Part model, mm, in its own coordinate system. Face numbers are marked on the shaded views. A direction names the side the tool comes from. Give positions to 0.01 mm unless a question says otherwise; leave off trailing zeros. Write each loop counter-clockwise with the first axis right and the second up, starting at its lowest first coordinate (ties: lowest second). Pieces come first, ordered by that corner, then holes. Notation, with made-up numbers: M 35,8 L 81,8 A8 cw 81,16 Z; hole C 54,83 d11. An arc over 180 degrees is marked long. Use a Markdown table: item, result.
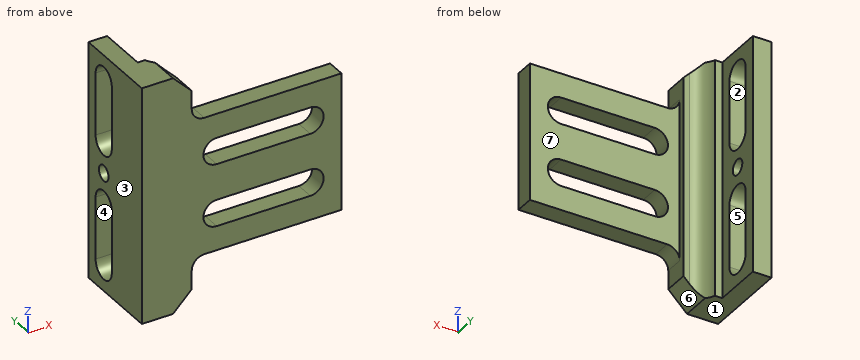
```python
from build123d import *

# Parameters (mm, degrees)
BASESTEELANGLE_DEPTH    = 60.325
CUT_EXTRUDE1_DEPTH      = 1
CUT_EXTRUDE1_DEPTH_BACK = 121.65
CUT_EXTRUDE3_DEPTH      = 13.7
SKETCH5_W               = 76.2
SKETCH5_H               = 6.35
CUT_EXTRUDE4_DEPTH      = 121.65
SKETCH6_W               = 9.525
SKETCH6_H               = 28.575
CUT_EXTRUDE5_DEPTH      = 121.65
CUT_EXTRUDE6_DEPTH      = 10.525
F_3_8_16_TAPPED_HOLE1_D = 7.9375
SKETCH11_W              = 25.4
SKETCH11_H              = 9.525
CUT_EXTRUDE8_DEPTH      = 76.2
FILLET2_R               = 6.35
CHAMFER3_SIZE           = 9.525


with BuildPart() as part:
    # Sketch1 → BaseSteelAngle (new body, symmetric)
    with BuildSketch(Plane.XY):
        with BuildLine():
            Line((0, 0), (0, 101.6))
            Line((0, 101.6), (3.18008, 101.6))
            ThreePointArc((3.18008, 101.6), (9.911679988, 98.811679988), (12.7, 92.08008))
            Line((12.7, 92.08008), (12.7, 22.225))
            ThreePointArc((12.7, 22.225), (15.489807909, 15.489807909), (22.225, 12.7))
            Line((22.225, 12.7), (101.6, 12.7))
            Line((101.6, 12.7), (101.6, 0))
            Line((101.6, 0), (0, 0))
        make_face()
    extrude(amount=BASESTEELANGLE_DEPTH, both=True)

    # Sketch2 → Cut-Extrude1 (cut, two sides)
    with BuildSketch(Plane.XY.offset(60.325)) as cut_extrude1_sk:
        Polygon((-254.455417258, 44.45), (-4.112271749, 44.45), (18.408340367, 44.45), (268.751485876, 44.45), (268.751485876, 545.136291018), (-254.455417258, 545.136291018), align=None)
    extrude(amount=CUT_EXTRUDE1_DEPTH, mode=Mode.SUBTRACT)
    extrude(cut_extrude1_sk.sketch, amount=-CUT_EXTRUDE1_DEPTH_BACK, mode=Mode.SUBTRACT)

    # Sketch4 → Cut-Extrude3 (cut, through all)
    with BuildSketch(Plane(origin=(78.166939161, 12.7, 45.281727152), x_dir=(0, 0, 1), z_dir=(0, 1, 0))):
        with BuildLine():
            Line((-67.902967152, 7.558060839), (-67.902967152, -40.066939161))
            ThreePointArc((-67.902967152, -40.066939161), (-61.156727152, -46.813179161), (-54.410487152, -40.066939161))
            Line((-54.410487152, -40.066939161), (-54.410487152, 7.558060839))
            ThreePointArc((-54.410487152, 7.558060839), (-61.156727152, 14.304300839), (-67.902967152, 7.558060839))
        make_face()
    cut_extrude3 = extrude(amount=-CUT_EXTRUDE3_DEPTH, mode=Mode.SUBTRACT)

    # Mirror1: Cut-Extrude3 across plane
    add(cut_extrude3.mirror(Plane.XY), mode=Mode.SUBTRACT)

    # Sketch5 → Cut-Extrude4 (cut, through all)
    with BuildSketch(Plane(origin=(0, 0, -60.325), x_dir=(-1, 0, 0), z_dir=(0, 0, -1))):
        with Locations((-63.5, 12.7)):
            Rectangle(SKETCH5_W, SKETCH5_H)
    extrude(amount=-CUT_EXTRUDE4_DEPTH, mode=Mode.SUBTRACT)

    # Sketch6 → Cut-Extrude5 (cut, through all)
    with BuildSketch(Plane(origin=(0, 0, -60.325), x_dir=(-1, 0, 0), z_dir=(0, 0, -1))):
        with Locations((-14.2875, 33.3375)):
            Rectangle(SKETCH6_W, SKETCH6_H)
    extrude(amount=-CUT_EXTRUDE5_DEPTH, mode=Mode.SUBTRACT)

    # Sketch7 → Cut-Extrude6 (cut, through all)
    with BuildSketch(Plane(origin=(9.525, 0, 0), x_dir=(0, 0, -1), z_dir=(1, 0, 0))):
        with BuildLine():
            Line((15.875, 25.003125), (47.625, 25.003125))
            ThreePointArc((47.625, 25.003125), (54.371875, 31.75), (47.625, 38.496875))
            Line((47.625, 38.496875), (15.875, 38.496875))
            ThreePointArc((15.875, 38.496875), (9.128125, 31.75), (15.875, 25.003125))
        make_face()
    cut_extrude6 = extrude(amount=-CUT_EXTRUDE6_DEPTH, mode=Mode.SUBTRACT)

    # Mirror2: Cut-Extrude6 across plane
    add(cut_extrude6.mirror(Plane.XY), mode=Mode.SUBTRACT)

    # 3/8-16 Tapped Hole1 (through all)
    with Locations(Plane(origin=(9.525, 0, 0), x_dir=(0, 0, -1), z_dir=(1, 0, 0))):
        with Locations((0, 31.75)):
            Hole(F_3_8_16_TAPPED_HOLE1_D / 2)

    # Sketch11 → Cut-Extrude8 (cut)
    with BuildSketch(Plane(origin=(101.6, 0, 0), x_dir=(0, 0, -1), z_dir=(1, 0, 0))):
        with Locations((47.625, 4.7625)):
            Rectangle(SKETCH11_W, SKETCH11_H)
        with Locations((-47.625, 4.7625)):
            Rectangle(SKETCH11_W, SKETCH11_H)
    extrude(amount=-CUT_EXTRUDE8_DEPTH, mode=Mode.SUBTRACT)

    # Fillet2
    fillet2_edges = [part.edges().sort_by_distance(p)[0] for p in [
        (25.4, 4.7625, -34.925),
        (25.4, 4.7625, 34.925),
    ]]
    fillet(fillet2_edges, radius=FILLET2_R)

    # Chamfer3
    chamfer3_edges = [part.edges().sort_by_distance(p)[0] for p in [
        (25.4, 6.35, 60.325),
        (25.4, 6.35, -60.325),
    ]]
    chamfer(chamfer3_edges, length=CHAMFER3_SIZE)


solid = part.part
```
1. Drill centre lines: L1, parallel to Z at x = 79, y = 7.5 (3 decimals); L2, parallel to Y at x = 3, z = 0; L3, parallel to Y at x = 8.5, z = 32.5. Where is each one in solid material? Low to high.
Findings below:
| item | result |
|---|---|
| L1 | -34.925 to -22.621, -9.129 to 9.129, 22.621 to 34.925 |
| L2 | 0 to 27.78, 35.72 to 44.45 |
| L3 | 0 to 25, 38.5 to 44.45 |
2. Cut at D-D, the plane z = 21. Give the cut face in (x, y) (3 decimals).
Findings below:
| item | result |
|---|---|
| outline | M 0,0 L 33.713,0 L 33.713,9.525 L 25.4,9.525 L 25.4,12.7 L 22.225,12.7 A9.525 cw 13.245,19.05 L 9.525,19.05 L 9.525,25.003 L 0,25.003 Z; M 0,38.497 L 9.525,38.497 L 9.525,44.45 L 0,44.45 Z; M 90.112,0 L 101.6,0 L 101.6,9.525 L 90.112,9.525 Z |
3. Cut at C-C, the plane y = 31.75. Give the cut face in (x, z) (3 decimals).
Findings below:
| item | result |
|---|---|
| outline | M 0,-60.325 L 9.525,-60.325 L 9.525,-54.372 L 0,-54.372 Z; M 0,-9.128 L 9.525,-9.128 L 9.525,-3.969 L 0,-3.969 Z; M 0,3.969 L 9.525,3.969 L 9.525,9.128 L 0,9.128 Z; M 0,54.372 L 9.525,54.372 L 9.525,60.325 L 0,60.325 Z |
4. Tool access for the marked faces 5, 6 and 7: list every direction of +Z, -Z, +X, -X, +Y, -Y with a clear straight run to the whole face (end or side of a thin tool).
Findings below:
| item | result |
|---|---|
| face 5 | +X, -X |
| face 6 | -Z, +X, +Y, -Y |
| face 7 | +Z, -Z, +X, +Y |
5. Two-plate mould, pull along Z, no slides. Class the marked faces 1, 2, 3 and 4: released by +Z, released by -Z, zero draft, split by the parting line, or undercut.
Findings below:
| item | result |
|---|---|
| face 1 | released by -Z |
| face 2 | undercut |
| face 3 | zero draft |
| face 4 | undercut |
6. Drop flat-ended pins along their axis: P1, Ø3, axis at x = 60.5, y = 5.5, coming from the +Z side (3 decimals); P2, Ø5, axis at x = 22.5, y = 13.5, coming from the -Z side; P3, Ø3, axis at x = 21.5, z = -46, coming from the +Y side. Give the stop position or say it passes through.
Findings below:
| item | result |
|---|---|
| P1 | z = 34.925 |
| P2 | z = -56.14 |
| P3 | y = 12.96 |
7. Cut at A-A, the plane z = 45.5. Give the cut face in (x, y) (3 decimals), then the cut area to 3 significant figures.
Findings below:
| item | result |
|---|---|
| outline | M 0,0 L 25.4,0 L 25.4,12.7 L 22.225,12.7 A9.525 cw 13.245,19.05 L 9.525,19.05 L 9.525,25.003 L 0,25.003 Z; M 0,38.497 L 9.525,38.497 L 9.525,44.45 L 0,44.45 Z |
| area | 536 mm2 |
8. Cut at B-B, the plane x = 83.5. Give the cut face in (y, z) (3 decimals).
Findings below:
| item | result |
|---|---|
| outline | M 0,-34.925 L 9.525,-34.925 L 9.525,-22.621 L 0,-22.621 Z; M 0,-9.129 L 9.525,-9.129 L 9.525,9.129 L 0,9.129 Z; M 0,22.621 L 9.525,22.621 L 9.525,34.925 L 0,34.925 Z |
